```python
from build123d import *

# Parameters (mm, degrees)
EXTRUDE_1_DEPTH     = 180
SKETCH_2_R          = 70
CUT_EXTRUDE_1_DEPTH = 180


with BuildPart() as part:
    # 草图1 → 凸台-拉伸1 (new body)
    with BuildSketch(Plane(origin=(0, 0, 0), x_dir=(1, 0, 0), z_dir=(0, 1, 0))):
        Polygon((0, 0), (43.3, 0), (43.3, -10), (8, -10), (8, -300), (0, -300), align=None)
    extrude(amount=EXTRUDE_1_DEPTH)

    # 草图2 → 切除-拉伸1 (cut)
    with BuildSketch(Plane(origin=(8, 0, 0), x_dir=(0, 0, -1), z_dir=(1, 0, 0))):
        with Locations((-90, 90)):
            Circle(SKETCH_2_R)
        with BuildLine():
            Line((-90, 0), (-300, 0))
            Line((-300, 0), (-300, 180))
            Line((-300, 180), (-90, 180))
            ThreePointArc((-90, 180), (-180, 90), (-90, 0))
        make_face()
    extrude(amount=-CUT_EXTRUDE_1_DEPTH, mode=Mode.SUBTRACT)


solid = part.part
```
Design review of the part built by this model. Coordinates are the model's own, in mm. A direction names the side the tool comes from. Give positions to 0.01 mm unless a question says otherwise; leave off trailing zeros. Order: outer loops, then holes, each group sorted by start corner. A loop starts at its lowest first (then second) coordinate and runs counter-clockwise, first axis right, second up. Notation, with made-up numbers: (-34, 18.25) - (-12, 18.25) arc R21 ccw to (-12, 23.25) - close; hole circle Ø8 at (23.5, 69). An arc over 180 degrees is marked (long way). Use a Markdown table: item, result. Add a question column.
(1) Add section B-B on z = 51.5. Give the boundary of the cut face in (x, y).
(2) Clearance check with a flat-ended pin moving along its axis: P1, Ø6, axis at x = 33, y = 134.5, coming from the +Z side. State where the tip first meets the part, or that it passes through.
(3) Add section D-D on z = 96.5. Give the boundary of the cut face in (x, y), then the cut area to 3 significant figures.
(4) Wall thickness on probe 1 along Y at (x, z) = (5, 90); probe 2 along Z at (x, y) = (16, 149); probe 3 along X at (y, z) = (18.5, 65.5): over which ranges is each line inside the solid? List them lowest first. Write a range as [from, to].
(5) Machinability: for faces 5 (the face through (7, 180, 31)), 6 (the face through (26, 89, 10)), which of the approach directions +Z, -Z, +X, -X, +Y, -Y give a long, thin tool a straight path to every point of the face, cutting with its end or side? Answer none if there is none.
(6) Add section A-A on y = 90. Give the boundary of the cut face in (x, z), then the cut area to 3 significant figures.
(7) Add section C-C on x = 32.5. Give the boundary of the cut face in (y, z), then the cut area to 3 significant figures.
(8) Mouldability with a two-part tool opening along Z and no side actions: class faces 1 (the face through (7, 0, 31)), 2 (the face through (4.056, 159.404, 99.113)), 3 (the face through (4.06, 91.98, 179.98)), 4 (the face through (21, 89, 0)) as +Z half, -Z half, draft (parallel to the pull), parting line (faces both ways), or undercut.
Report:
| question | item | result |
|---|---|---|
| 1 | outline | (0, 0) - (8, 0) - (8, 31.54) - (0, 31.54) - close; (0, 148.46) - (8, 148.46) - (8, 180) - (0, 180) - close |
| 2 | P1 | stops at z = 10 |
| 3 | outline | (0, 0.24) - (8, 0.24) - (8, 20.3) - (0, 20.3) - close; (0, 159.7) - (8, 159.7) - (8, 179.76) - (0, 179.76) - close |
| 3 | area | 321 mm² |
| 4 | probe 1 | y = [0, 20], [160, 180] |
| 4 | probe 2 | z = [0, 10] |
| 4 | probe 3 | x = [0, 8] |
| 5 | face 5 | +Z, -Z, +X, -X, +Y |
| 5 | face 6 | +Z, +X, +Y, -Y |
| 6 | outline | (0, 0) - (43.3, 0) - (43.3, 10) - (8, 10) - (8, 20) - (0, 20) - close; (0, 160) - (8, 160) - (8, 180) - (0, 180) - close |
| 6 | area | 673 mm² |
| 7 | outline | (0, 0) - (180, 0) - (180, 10) - (0, 10) - close |
| 7 | area | 1,800 mm² |
| 8 | face 1 | draft |
| 8 | face 2 | undercut |
| 8 | face 3 | +Z half |
| 8 | face 4 | -Z half |
